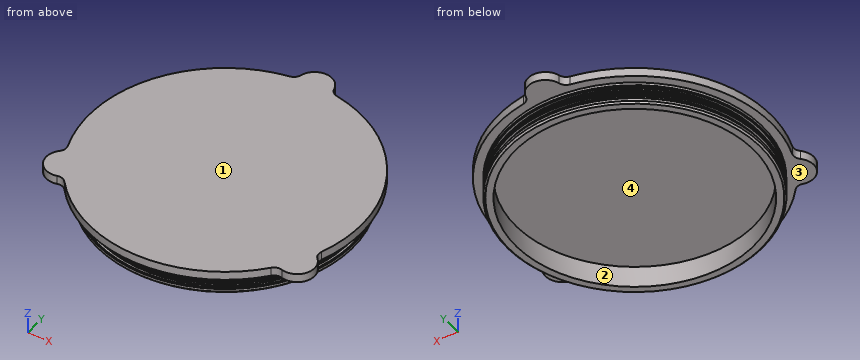
from build123d import *

# Parameters (mm, degrees)
SKETCH1_R          = 100.0125
EXTRUDE1_DEPTH     = 6.35
SKETCH2_R          = 93.6625
EXTRUDE2_DEPTH     = 15.875
SKETCH3_R          = 87.3125
CUT_EXTRUDE1_DEPTH = 15.875
SKETCH4_W          = 3.175
SKETCH4_H          = 2.54
CHAMFER1_SIZE      = 1.27
EXTRUDE3_DEPTH     = 6.35
CHAMFER2_SIZE      = 0.635
FILLET1_R          = 6.35


with BuildPart() as part:
    # Sketch1 → Extrude1 (new body)
    with BuildSketch(Plane.XY):
        Circle(SKETCH1_R)
    extrude(amount=EXTRUDE1_DEPTH)

    # Sketch2 → Extrude2 (add)
    with BuildSketch(Plane(origin=(0, 0, 0), x_dir=(-1, 0, 0), z_dir=(0, 0, -1))):
        Circle(SKETCH2_R)
    extrude(amount=EXTRUDE2_DEPTH)

    # Sketch3 → Cut-Extrude1 (cut)
    with BuildSketch(Plane(origin=(0, 0, -15.875), x_dir=(-1, 0, 0), z_dir=(0, 0, -1))):
        Circle(SKETCH3_R)
    extrude(amount=-CUT_EXTRUDE1_DEPTH, mode=Mode.SUBTRACT)

    # Sketch4 → Cut-Revolve1 (revolve, cut)
    with BuildSketch(Plane(origin=(0, 0, 0), x_dir=(0, 0, -1), z_dir=(1, 0, 0))):
        with Locations((4.395911794, 92.3925)):
            Rectangle(SKETCH4_W, SKETCH4_H)
        with Locations((10.251990741, 92.3925)):
            Rectangle(SKETCH4_W, SKETCH4_H)
    revolve(axis=Axis((0, 0, 0), (0, 0, -1)), mode=Mode.SUBTRACT)

    # Chamfer1
    chamfer1_edges = [part.edges().sort_by_distance(p)[0] for p in [
        (93.6625, 0, -15.875),
    ]]
    chamfer(chamfer1_edges, length=CHAMFER1_SIZE)

    # Sketch8 → Extrude3 (add)
    with BuildSketch(Plane.XY.offset(6.35)):
        with BuildLine():
            ThreePointArc((-12.674375762, 99.206150794), (0, 112.7125), (12.674375762, 99.206150794))
            ThreePointArc((12.674375762, 99.206150794), (0, 100.0125), (-12.674375762, 99.206150794))
        make_face()
        with BuildLine():
            ThreePointArc((92.25223468, -38.62674401), (97.611888324, -56.35625), (79.577858918, -60.579406784))
            ThreePointArc((79.577858918, -60.579406784), (86.613365696, -50.00625), (92.25223468, -38.62674401))
        make_face()
        with BuildLine():
            ThreePointArc((-92.25223468, -38.62674401), (-97.611888324, -56.35625), (-79.577858918, -60.579406784))
            ThreePointArc((-79.577858918, -60.579406784), (-86.613365696, -50.00625), (-92.25223468, -38.62674401))
        make_face()
    extrude(amount=-EXTRUDE3_DEPTH)

    # Chamfer2
    chamfer2_edges = [part.edges().sort_by_distance(p)[0] for p in [
        (93.6625, 0, -2.808411794),
        (93.6625, 0, -5.983411794),
        (93.6625, 0, -8.664490741),
        (93.6625, 0, -11.839490741),
    ]]
    chamfer(chamfer2_edges, length=CHAMFER2_SIZE)

    # Fillet1
    fillet1_edges = [part.edges().sort_by_distance(p)[0] for p in [
        (12.674375762, 99.206150794, 3.175),
        (-12.674375762, 99.206150794, 3.175),
        (79.577858918, -60.579406784, 3.175),
        (92.25223468, -38.62674401, 3.175),
        (-92.25223468, -38.62674401, 3.175),
        (-79.577858918, -60.579406784, 3.175),
    ]]
    fillet(fillet1_edges, radius=FILLET1_R)


solid = part.part
Geometry check sheet. Reference: the model listing, model coordinates, mm. Face numbers are marked on the shaded views. A direction names the side the tool comes from. Give positions to 0.01 mm unless a question says otherwise; leave off trailing zeros.
(1) Release check for a two-part mould opening along X. For the marked faces 3 and 4 record: released by +X, released by -X, zero draft, split by the parting line, or undercut.
From the geometry:
face 3: zero draft
face 4: undercut
(2) Thickness scan on L1, parallel to Y at x = 0, z = -7.25; L2, parallel to Z at x = 62, y = -77; L3, parallel to Y at x = -31.5, z = -9. Record the ranges inside material, lowest first.
From the geometry:
L1: y = -93.66 to -87.31, 87.31 to 93.66
L2: z = 0 to 6.35
L3: y = -85.5 to -81.43, 81.43 to 85.5
(3) Depth check by flat-ended pin: pin 1 Ø12 at (x, y) = (-43.5, 33) entering from -Z; pin 2 Ø10 at (x, z) = (-1, -11.5) entering from -Y; pin 3 Ø2 at (y, z) = (-40.5, -9.5) entering from -X. Enter the tip coordinate at first touch or a pass-through.
From the geometry:
pin 1: stops at z = 0
pin 2: stops at y = -93.66
pin 3: stops at x = -84.03
(4) Set-up check for the marked faces 1 and 2: record each of +Z, -Z, +X, -X, +Y, -Y from which the full face is reachable in a straight line by a thin tool's end or side.
From the geometry:
face 1: +Z, +X, -X, +Y, -Y
face 2: -Z
